Geometry check sheet. Reference: the model listing, model coordinates, mm. Face numbers are marked on the shaded views. A direction names the side the tool comes from. Round coordinates to 2 decimals unless told otherwise and drop trailing zeros. Order: outer loops, then holes, each group sorted by start corner. A loop starts at its lowest first (then second) coordinate and runs counter-clockwise, first axis right, second up.
```python
from build123d import *

# Parameters (mm, degrees)
SKETCH_1_R      = 11
EXTRUDE_1_DEPTH = 15
SKETCH_2_R      = 14.5
EXTRUDE_2_DEPTH = 11
SKETCH_3_W      = 6.140328376
SKETCH_3_H      = 29.814639278
EXTRUDE_3_DEPTH = 10


with BuildPart() as part:
    # 草图1 → 凸台-拉伸1 (new body)
    with BuildSketch(Plane.XY):
        Circle(SKETCH_1_R)
    extrude(amount=EXTRUDE_1_DEPTH)

    # 草图2 → 凸台-拉伸2 (add)
    with BuildSketch(Plane.XY.offset(15)):
        Circle(SKETCH_2_R)
    extrude(amount=EXTRUDE_2_DEPTH)

    # 草图3 → 凸台-拉伸3 (add)
    with BuildSketch(Plane.XY.offset(26)):
        Rectangle(SKETCH_3_W, SKETCH_3_H)
    extrude(amount=EXTRUDE_3_DEPTH)


solid = part.part
```
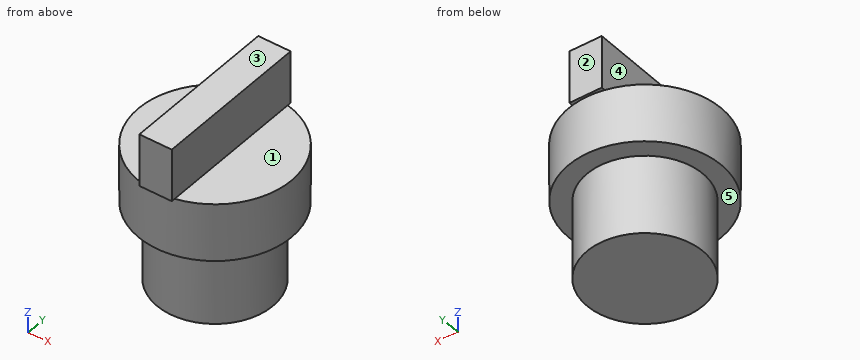
(1) Sectioned sample at C-C, the plane z = 5. Record the cut outline in (x, y), and give its area (3 significant figures).
Returned:
outline: circle Ø22 at (0, 0)
area: 380 mm2
(2) Sectioned sample at A-A, the plane x = 0. Record the cut outline in (y, z), and give its area (3 significant figures).
Returned:
outline: (-14.91, 26) - (-14.5, 26) - (-14.5, 15) - (-11, 15) - (-11, 0) - (11, 0) - (11, 15) - (14.5, 15) - (14.5, 26) - (14.91, 26) - (14.91, 36) - (-14.91, 36) - close
area: 947 mm2
(3) Depth check by flat-ended pin: P1, Ø8, axis at x = -3.5, y = 6.5, coming from the -Z side; P2, Ø8, axis at x = 9, z = 12, coming from the -Y side; P3, Ø6, axis at y = -5, z = 4, coming from the +X side; P4, Ø9, axis at x = 9.5, y = -2, coming from the +Z side. Enter the tip coordinate at first touch or a pass-through.
Returned:
P1: stops at z = 0
P2: stops at y = -13.03
P3: stops at x = 10.82
P4: stops at z = 26
(4) Material ranges on line 1 (Z direction, x = 4.75, y = 10.5); line 2 (Y direction, x = -0.5, z = 3.5); line 3 (Z direction, x = 5.25, y = -5.75), recorded low to high.
Returned:
line 1: z = 15 to 26
line 2: y = -10.99 to 10.99
line 3: z = 0 to 26
(5) Sectioned sample at B-B, the plane y = 0. Record the cut outline in (x, z).
Returned:
outline: (-14.5, 15) - (-11, 15) - (-11, 0) - (11, 0) - (11, 15) - (14.5, 15) - (14.5, 26) - (3.07, 26) - (3.07, 36) - (-3.07, 36) - (-3.07, 26) - (-14.5, 26) - close
(6) Sectioned sample at D-D, the plane x = -4.5. Record the cut outline in (y, z).
Returned:
outline: (-13.78, 15) - (-10.04, 15) - (-10.04, 0) - (10.04, 0) - (10.04, 15) - (13.78, 15) - (13.78, 26) - (-13.78, 26) - close
(7) Set-up check for the marked faces 1, 2, 3, 4 and 5: record each of +Z, -Z, +X, -X, +Y, -Y from which the full face is reachable in a straight line by a thin tool's end or side.
Returned:
face 1: +Z, +X, +Y, -Y
face 2: +Z, -Z, +X, -X, +Y
face 3: +Z, +X, -X, +Y, -Y
face 4: +Z, -X, +Y, -Y
face 5: -Z
